Build history of the part. All positions in model axes, mm. Give positions to 0.01 mm unless a question says otherwise; leave off trailing zeros. Order: outer loops, then holes, each group sorted by start corner. A loop starts at its lowest first (then second) coordinate and runs counter-clockwise, first axis right, second up. Notation, with made-up numbers: (-28, 52.5) - (-10, 52.5) arc R12 ccw to (-10, 67.5) - close; hole circle Ø6 at (6.25, -9). An arc over 180 degrees is marked (long way). Answer in a Markdown table with one row per item.
```python
from build123d import *

# Parameters (mm, degrees)
SKETCH_1_W          = 200
SKETCH_1_H          = 120
SKETCH_1_R          = 4
EXTRUDE_1_DEPTH     = 5
SKETCH_2_W          = 20
SKETCH_2_H          = 25
SKETCH_2_R          = 2.05
EXTRUDE_2_DEPTH     = 5
EXTRUDE_3_DEPTH     = 5
SKETCH_4_W          = 10.1
SKETCH_4_H          = 15.1
CUT_EXTRUDE_1_DEPTH = 312.84932259
SKETCH_5_W          = 5
SKETCH_5_H          = 20
EXTRUDE_4_DEPTH     = 5


with BuildPart() as part:
    # 草圖1 → 填料-伸長1 (new body)
    with BuildSketch(Plane(origin=(0, 0, 0), x_dir=(0, 0, -1), z_dir=(1, 0, 0))):
        Rectangle(SKETCH_1_W, SKETCH_1_H)
        with Locations((-10, 40)):
            Circle(SKETCH_1_R, mode=Mode.SUBTRACT)
    extrude(amount=EXTRUDE_1_DEPTH)

    # 草圖2 → 填料-伸長2 (add)
    # profile 1 of 3: a face of its own
    with BuildSketch(Plane(origin=(5, 0, 0), x_dir=(0, 0, -1), z_dir=(1, 0, 0))):
        with Locations((-60, -72.5)):
            Rectangle(SKETCH_2_W, SKETCH_2_H)
        with Locations((-60, -75)):
            Circle(SKETCH_2_R, mode=Mode.SUBTRACT)
    # profile 2 of 3: a face of its own
    with BuildSketch(Plane(origin=(5, 0, 0), x_dir=(0, 0, -1), z_dir=(1, 0, 0))):
        with Locations((0, -72.5)):
            Rectangle(SKETCH_2_W, SKETCH_2_H)
        with Locations((0, -75)):
            Circle(SKETCH_2_R, mode=Mode.SUBTRACT)
    # profile 3 of 3: a face of its own
    with BuildSketch(Plane(origin=(5, 0, 0), x_dir=(0, 0, -1), z_dir=(1, 0, 0))):
        with Locations((60, -72.5)):
            Rectangle(SKETCH_2_W, SKETCH_2_H)
        with Locations((60, -75)):
            Circle(SKETCH_2_R, mode=Mode.SUBTRACT)
    extrude(amount=-EXTRUDE_2_DEPTH)

    # 草圖3 → 填料-伸長3 (add)
    with BuildSketch(Plane(origin=(5, 0, 0), x_dir=(0, 0, -1), z_dir=(1, 0, 0))):
        Polygon((-100, 60), (-300, 60), (-300, 30), (-130, -60), (-100, -60), align=None)
        Polygon((-130, 30), (-130, -26.055204597), (-235.882053128, 30), align=None, mode=Mode.SUBTRACT)
    extrude(amount=-EXTRUDE_3_DEPTH)

    # 草圖4 → 除料-伸長1 (cut, through all)
    with BuildSketch(Plane(origin=(5, 0, 0), x_dir=(0, 0, -1), z_dir=(1, 0, 0))):
        with Locations((-88.95, -17.35)):
            Rectangle(SKETCH_4_W, SKETCH_4_H)
        with Locations((-88.95, -47.45)):
            Rectangle(SKETCH_4_W, SKETCH_4_H)
    extrude(amount=-CUT_EXTRUDE_1_DEPTH, mode=Mode.SUBTRACT)

    # 草圖5 → 填料-伸長4 (add)
    with BuildSketch(Plane(origin=(0, 60, 0), x_dir=(1, 0, 0), z_dir=(0, 1, 0))):
        with Locations((2.5, -160)):
            Rectangle(SKETCH_5_W, SKETCH_5_H)
        with Locations((2.5, -240)):
            Rectangle(SKETCH_5_W, SKETCH_5_H)
    extrude(amount=EXTRUDE_4_DEPTH)


solid = part.part
```
1. Probe line 1 (Y direction, x = 3.2, z = -60); line 2 (Y direction, x = 2.3, z = 192); line 3 (Z direction, x = 4.4, y = 10.5). List the from-to ranges inside material, lowest first.
Check result:
| item | result |
|---|---|
| line 1 | y = -85 to -77.05, -72.95 to 60 |
| line 2 | y = -27.18 to 6.77, 30 to 60 |
| line 3 | z = -100 to 130, 199.05 to 263.17 |
2. Cut at A-A on z = 214.5. Write the cut outline in (x, y).
Check result:
| item | result |
|---|---|
| outline | (0, -15.26) - (5, -15.26) - (5, 18.68) - (0, 18.68) - close; (0, 30) - (5, 30) - (5, 60) - (0, 60) - close |
3. Cut at B-B on x = 3.35. Count the separate pieces of the cut face and the enclosed holes in it, and give its area (3 significant figures).
Check result:
| item | result |
|---|---|
| separate pieces | 1 |
| enclosed holes | 7 |
| area | 38,700 mm² |
4. Cut at C-C on z = 24.5. Write the cut outline in (x, y), and give its area (3 significant figures).
Check result:
| item | result |
|---|---|
| outline | (0, -60) - (5, -60) - (5, 60) - (0, 60) - close |
| area | 600 mm² |
5. Drop flat-ended pins along their axis: P1, Ø3, axis at x = 2.5, z = 113, coming from the -Y side; P2, Ø2.5, axis at x = 3, z = 86.5, coming from the +Y side; P3, Ø2.5, axis at y = -75, z = 60, coming from the -X side; P4, Ø1, axis at x = 2.5, y = -36.5, coming from the +Z side. Give the stop position or say it passes through.
Check result:
| item | result |
|---|---|
| P1 | stops at y = -60 |
| P2 | stops at y = 60 |
| P3 | passes through |
| P4 | stops at z = 175.33 |
6. Two-plate mould, pull along Y, no slides. Class faces 1 (the face through (2.54, 1.58, 182.2)), 2 (the face through (0, 8, 58)), 3 (the face through (2.54, -14.37, 216.19)): +Y half, -Y half, draft (parallel to the pull), parting line (faces both ways), or undercut.
Check result:
| item | result |
|---|---|
| face 1 | undercut |
| face 2 | draft |
| face 3 | -Y half |
